Autodesk Fusion 360 part; units mm, degrees
sketch "草图1" plane through (0, 0, 0) normal (1, 0, 0) x (0, 0, -1)
cylinder "圆柱体基本要素1" add diameter 8 height 100 placed x (1, 0, 0) y (0, 0, -1) z (0, 1, 0) at (0, 0, 0) makes body 1
sketch "草图3" plane through (0, 0, 0) normal (0, 0, 1) x (1, 0, 0)
  line L0 (0, 0) -> (4, 0)
  line L1 (4, 0) -> (0, -10)
  line L2 (0, -10) -> (0, 0)
  dimension "d3" = 4
sketch "草图4" plane through (0, 0, 0) normal (0, 0, 1) x (1, 0, 0)
  line L0 (0, 0) -> (4, 0)
  line L1 (0, 0) -> (0, -15)
  line L2 (0, -15) -> (4, 0)
  dimension "d5" = 4
  dimension "d6" = 15
revolve "旋转2" add sketch "草图4" angle 360 about axis through (0, 0, 0) along (0, -1, 0) separate body makes body 2
combine "合并1" operation add target body 2 tool bodies 1
Geometry: final body of the model. Coordinates: model frame, mm. Coordinates: 2 decimals unless noted, no trailing zeros. Order: outer loops, then holes, each group sorted by start corner. A loop starts at its lowest first (then second) coordinate and runs counter-clockwise, first axis right, second up.
1) Section A-A (y = 11). Return loops of the section in (x, z), then the cut area to 3 significant figures.
Result sheet:
outline: circle Ø8 at (0, 0)
area: 50.3 mm2
2) First-contact query: P1, Ø2, axis at y = 12, z = -2.5, coming from the +X side; P2, Ø3, axis at x = 2.5, y = 70.5, coming from the +Z side. Flat tips, straight axial feed; report the tip coordinate or a pass-through.
Result sheet:
P1: stops at x = 3.71
P2: stops at z = 3.87
3) Ray query, probe 1 along Z at (x, y) = (-0.25, 50.5); probe 2 along X at (y, z) = (24, -3); probe 3 along X at (y, z) = (65, 1.25). Return the intervals inside material, ascending.
Result sheet:
probe 1: z = -3.99 to 3.99
probe 2: x = -2.65 to 2.65
probe 3: x = -3.8 to 3.8
